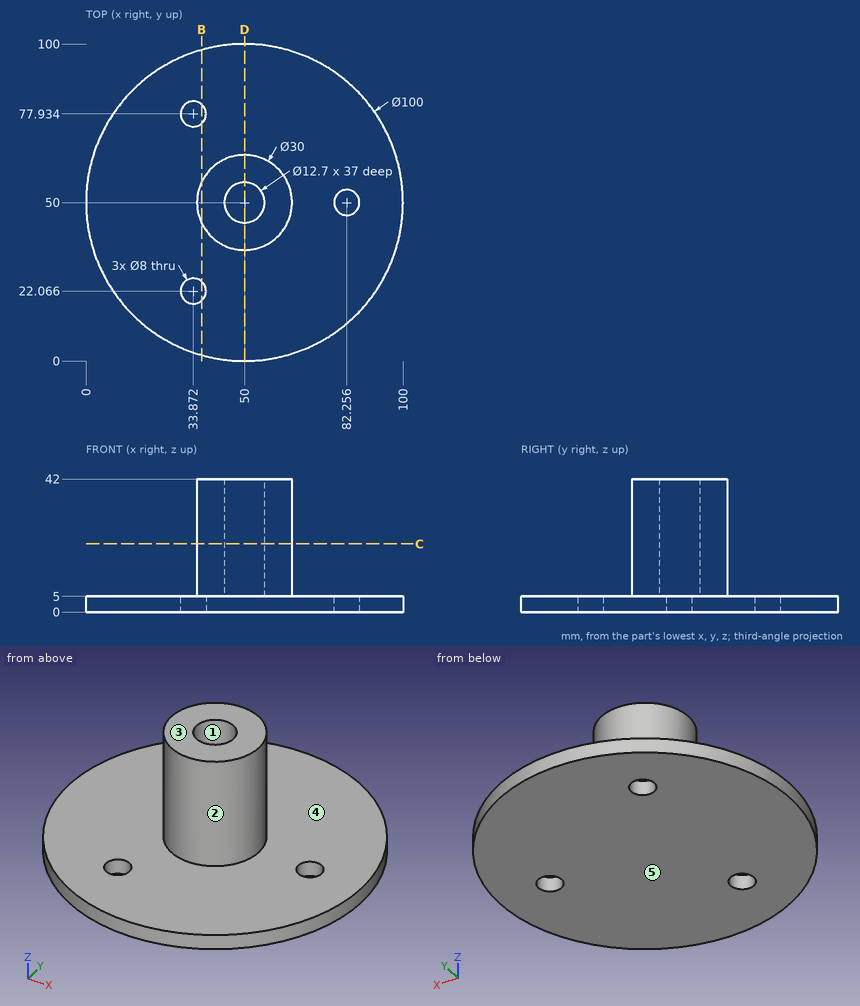
Here's the drawing with two shaded views (mm, measured from the low corner). I have some questions. A direction names the side the tool comes from. Coordinates: 2 decimals unless noted, no trailing zeros. Loops run counter-clockwise (first coordinate to the right, second up) from the corner with the lowest first, then second, coordinate; pieces in that order, holes last. Notation, with made-up numbers: (86, -15.75) -> (124, -15.75) arc R23 cw to (124, -0.75) -> close; hole circle Ø1 at (5.25, -26). An arc over 180 degrees is marked (long way). Answer in a Markdown table with one row per item.
(1) Thinking about a two-plate mould opening in X: for the marked faces 1, 2 and 3, which applies, released by +X, released by -X, zero draft, split by the parting line, or undercut?
Results found:
| item | result |
|---|---|
| face 1 | undercut |
| face 2 | split by the parting line |
| face 3 | zero draft |
(2) Imagine slicing it at C-C (z = 21.5). List the corners of the cut face in (x, y) for me.
Results found:
| item | result |
|---|---|
| outline | circle Ø30 at (50, 50); hole circle Ø12.7 at (50, 50) |
(3) Imagine slicing it at D-D (x = 50). List the corners of the cut face in (y, z) for me.
Results found:
| item | result |
|---|---|
| outline | (0, 0) -> (100, 0) -> (100, 5) -> (65, 5) -> (65, 42) -> (56.35, 42) -> (56.35, 5) -> (43.65, 5) -> (43.65, 42) -> (35, 42) -> (35, 5) -> (0, 5) -> close |
(4) Will these pins go through, and if not, where does the flat tip stop? pin 1 Ø6 at (y, z) = (48, 16) entering from -X; pin 2 Ø10.5 at (x, y) = (33.87, 22.07) entering from +Z; pin 3 Ø13 at (x, y) = (33.87, 77.93) entering from -Z; pin 4 Ø12 at (x, z) = (48, 13) entering from -Y.
Results found:
| item | result |
|---|---|
| pin 1 | stops at x = 35 |
| pin 2 | stops at z = 5 |
| pin 3 | stops at z = 0 |
| pin 4 | stops at y = 35 |
(5) For the marked faces 4 and 5, which set-ups out of +Z, -Z, +X, -X, +Y, -Y let a thin tool reach every point of the face, with its end or its side?
Results found:
| item | result |
|---|---|
| face 4 | +Z |
| face 5 | -Z, +X, -X, +Y, -Y |
(6) If I drill on probe 1 along Y at (x, z) = (49.5, 18); probe 2 along Z at (x, y) = (67, 66); probe 3 along Y at (x, z) = (48, 18) (1 decimal), over which ranges is the centre line in solid material (lowest first)?
Results found:
| item | result |
|---|---|
| probe 1 | y = 35.01 to 43.67, 56.33 to 64.99 |
| probe 2 | z = 0 to 5 |
| probe 3 | y = 35.1 to 44, 56 to 64.9 |
(7) Imagine slicing it at B-B (x = 36.5). List the corners of the cut face in (y, z) for me.
Results found:
| item | result |
|---|---|
| outline | (1.86, 0) -> (19.05, 0) -> (19.05, 5) -> (1.86, 5) -> close; (25.08, 0) -> (74.92, 0) -> (74.92, 5) -> (56.54, 5) -> (56.54, 42) -> (43.46, 42) -> (43.46, 5) -> (25.08, 5) -> close; (80.95, 0) -> (98.14, 0) -> (98.14, 5) -> (80.95, 5) -> close |
